Verification items for this drawing (mm, ordinates from the low corner). A direction names the side the tool comes from. Coordinates: 2 decimals unless noted, no trailing zeros. Loops run counter-clockwise (first coordinate to the right, second up) from the corner with the lowest first, then second, coordinate; pieces in that order, holes last. Notation, with made-up numbers: M -39.5,4.25 L -34.5,4.25 A13 cw -34.5,12.25 Z; hole C 81.5,28.25 d2. An arc over 180 degrees is marked long. Return JSON: item names as keys, results as strings.
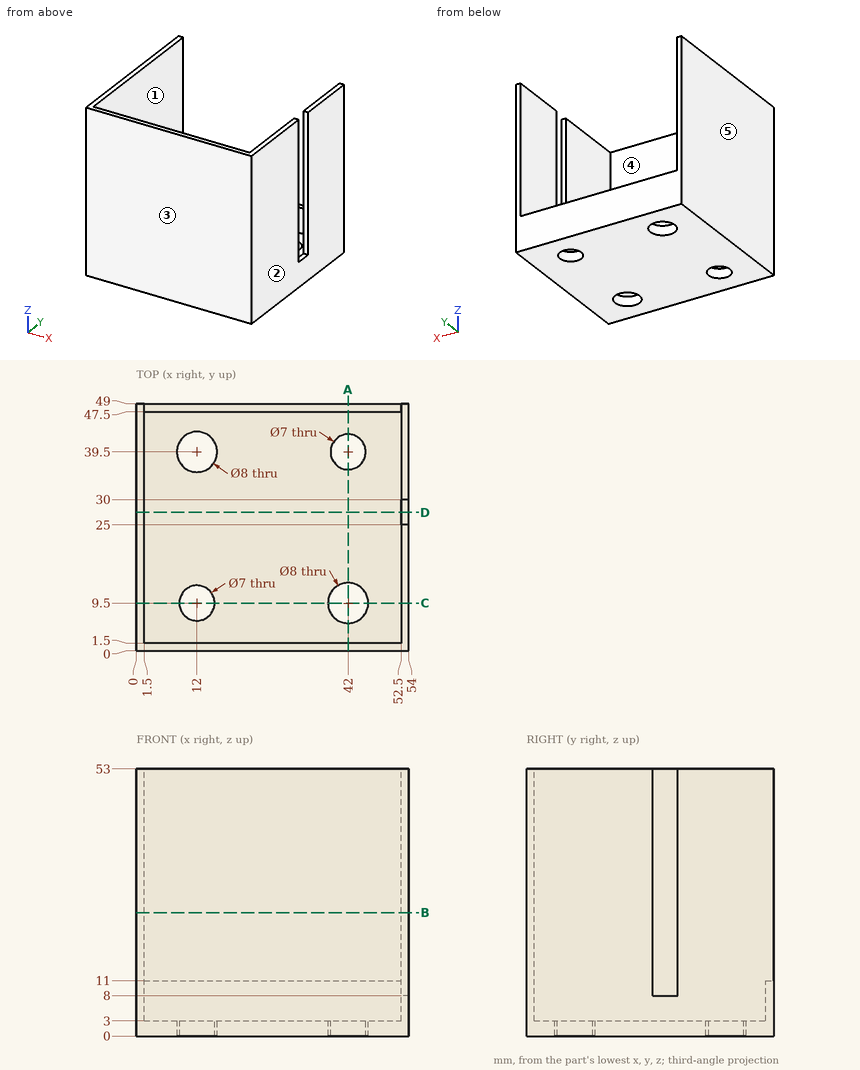
1) Section check B-B on z = 24.5. Record the cut outline in (x, y), then the cut area to 3 significant figures.
Answers:
{"outline": "M 0,0 L 54,0 L 54,25 L 52.5,25 L 52.5,1.5 L 1.5,1.5 L 1.5,49 L 0,49 Z; M 52.5,30 L 54,30 L 54,49 L 52.5,49 Z", "area": "216 mm²"}
2) Scan lines: line 1 along Y through (x, z) = (12, 1); line 2 along Y through (x, z) = (42, 0.8); line 3 along X through (y, z) = (6.5, 39). Record each from-to range of solid material in increasing order. Write a range as [from, to].
Answers:
{"line 1": "[0, 6], [13, 35.5], [43.5, 49]", "line 2": "[0, 5.5], [13.5, 36], [43, 49]", "line 3": "[0, 1.5], [52.5, 54]"}
3) Section check C-C on y = 9.5. Record the cut outline in (x, z), then the cut area to 3 significant figures.
Answers:
{"outline": "M 0,0 L 8.5,0 L 8.5,3 L 1.5,3 L 1.5,53 L 0,53 Z; M 15.5,0 L 38,0 L 38,3 L 15.5,3 Z; M 46,0 L 54,0 L 54,53 L 52.5,53 L 52.5,3 L 46,3 Z", "area": "267 mm²"}
4) Section check D-D on y = 27.5. Record the cut outline in (x, z).
Answers:
{"outline": "M 0,0 L 54,0 L 54,8 L 52.5,8 L 52.5,3 L 1.5,3 L 1.5,53 L 0,53 Z"}
5) Section check A-A on x = 42. Record the cut outline in (y, z), then the cut area to 3 significant figures.
Answers:
{"outline": "M 0,0 L 5.5,0 L 5.5,3 L 1.5,3 L 1.5,53 L 0,53 Z; M 13.5,0 L 36,0 L 36,3 L 13.5,3 Z; M 43,0 L 49,0 L 49,11 L 47.5,11 L 47.5,3 L 43,3 Z", "area": "189 mm²"}
6) Set-up check for the marked faces 1 and 2: record each of +Z, -Z, +X, -X, +Y, -Y from which the full face is reachable in a straight line by a thin tool's end or side.
Answers:
{"face 1": "+Z", "face 2": "+Z, -Z, +X, +Y, -Y"}
7) Draft check along Y on the marked faces 3, 4 and 5. Enter one of: +Y half, -Y half, draft (parallel to the pull), parting line (faces both ways), or undercut.
Answers:
{"face 3": "-Y half", "face 4": "undercut", "face 5": "draft"}
8) Go/stop test with flat-tipped pins: pin 1 Ø10 at (x, y) = (46.5, 15.5) entering from +Z; pin 2 Ø0.8 at (x, y) = (15.5, 48.5) entering from +Z; pin 3 Ø0.8 at (x, y) = (53.5, 27.5) entering from +Z. Record where each tip stops, or that it passes through.
Answers:
{"pin 1": "z = 3", "pin 2": "z = 11", "pin 3": "z = 8"}
